Read the model definition and answer for the solid it produces. Units are mm, in the model's axes. Face numbers are marked on the shaded views. A direction names the side the tool comes from. Coordinates: 2 decimals unless noted, no trailing zeros. Order: outer loops, then holes, each group sorted by start corner. A loop starts at its lowest first (then second) coordinate and runs counter-clockwise, first axis right, second up. Notation, with made-up numbers: (-31, -10) - (1, -10) arc R12 ccw to (1, -6) - close; hole circle Ø11 at (-0.5, -14.75). An arc over 180 degrees is marked (long way). Use one line per item in the form item = value.
```python
from build123d import *

# Parameters (mm, degrees)
SKETCH_1_R             = 11
SKETCH_1_R_2           = 1.75
EXTRUDE_1_DEPTH        = 3.6
SKETCH_2_R             = 5
SKETCH_2_R_2           = 4
EXTRUDE_1_2_DEPTH      = 10
EXTRUDE_1_2_DEPTH_BACK = 5.1
SKETCH_3_R             = 4
CUT_EXTRUDE_1_DEPTH    = 14.6


with BuildPart() as part:
    # Эскиз1 → Extrude 1 (new body)
    with BuildSketch(Plane.XY):
        Circle(SKETCH_1_R)
        with Locations((0, 8)):
            Circle(SKETCH_1_R_2, mode=Mode.SUBTRACT)
        with Locations((8, 0)):
            Circle(SKETCH_1_R_2, mode=Mode.SUBTRACT)
        with Locations((0, -8)):
            Circle(SKETCH_1_R_2, mode=Mode.SUBTRACT)
        with Locations((-8, 0)):
            Circle(SKETCH_1_R_2, mode=Mode.SUBTRACT)
    extrude(amount=EXTRUDE_1_DEPTH)

    # Эскиз2 → Extrude 1 2 (add, two sides)
    with BuildSketch(Plane.XY.offset(3.6)) as extrude_1_2_sk:
        Circle(SKETCH_2_R)
        Circle(SKETCH_2_R_2, mode=Mode.SUBTRACT)
    extrude(amount=EXTRUDE_1_2_DEPTH)
    extrude(extrude_1_2_sk.sketch, amount=-EXTRUDE_1_2_DEPTH_BACK)

    # Эскиз3 → Вырез-Вытянуть1 (cut, through all)
    with BuildSketch(Plane(origin=(0, 0, 0), x_dir=(-1, 0, 0), z_dir=(0, 0, -1))):
        Circle(SKETCH_3_R)
    extrude(amount=-CUT_EXTRUDE_1_DEPTH, mode=Mode.SUBTRACT)


solid = part.part
```
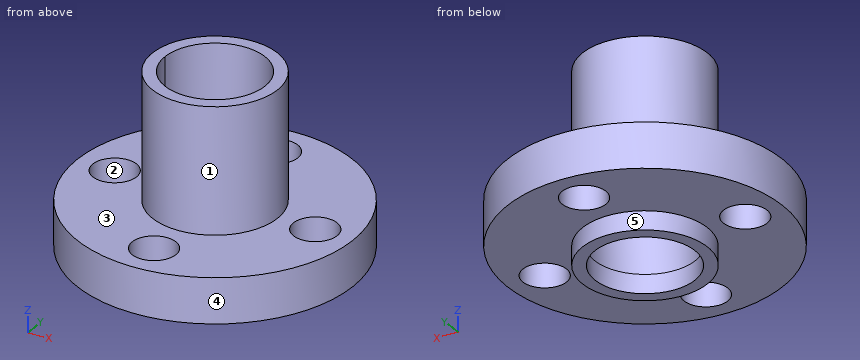
(1) Given pin 1 Ø3 at (x, y) = (8.5, 0.5) entering from +Z; pin 2 Ø1.5 at (x, z) = (1, 3.5) entering from +Y; pin 3 Ø3 at (x, z) = (-7.5, 4) entering from -Y, each flat-ended and moving along its own axis, determine where each tip first touches the part or whether it passes through.
Answer list:
pin_1 = 3.6
pin_2 = 11
pin_3 = -9.18
(2) Section A-A, the plane x = 0 is taken. Write down the section's boundary in (y, z), then the cut area to 3 significant figures.
Answer list:
outline = (-11, 0) - (-9.75, 0) - (-9.75, 3.6) - (-11, 3.6) - close; (-6.25, 0) - (-5, 0) - (-5, -1.5) - (-4, -1.5) - (-4, 13.6) - (-5, 13.6) - (-5, 3.6) - (-6.25, 3.6) - close; (4, -1.5) - (5, -1.5) - (5, 0) - (6.25, 0) - (6.25, 3.6) - (5, 3.6) - (5, 13.6) - (4, 13.6) - close; (9.75, 0) - (11, 0) - (11, 3.6) - (9.75, 3.6) - close
area = 48.2 mm2
(3) Section C-C, the plane y = -8.5 is taken. Write down the section's boundary in (x, z), then the cut area to 3 significant figures.
Answer list:
outline = (-6.98, 0) - (-1.68, 0) - (-1.68, 3.6) - (-6.98, 3.6) - close; (1.68, 0) - (6.98, 0) - (6.98, 3.6) - (1.68, 3.6) - close
area = 38.2 mm2
(4) Straight lines are drawn through the part: L1, parallel to Y at x = 0, z = 1.4; L2, parallel to Y at x = 0, z = -1.1; L3, parallel to X at y = -2, z = 8.25. For each, find the intervals that lie inside material, in ascending order.
Answer list:
L1 = -11 to -9.75, -6.25 to -4, 4 to 6.25, 9.75 to 11
L2 = -5 to -4, 4 to 5
L3 = -4.58 to -3.46, 3.46 to 4.58
(5) Which of the six approach directions +Z, -Z, +X, -X, +Y, -Y give full straight-line access (tool end or side, diameter ignored) to the marked faces 4 and 5?
Answer list:
face_4 = +Z, -Z
face_5 = -Z
(6) Section B-B, the plane z = 6.75 is taken. Write down the section's boundary in (x, y).
Answer list:
outline = circle Ø10 at (0, 0); hole circle Ø8 at (0, 0)
(7) Section D-D, the plane x = -8 is taken. Write down the section's boundary in (y, z), then the cut area to 3 significant figures.
Answer list:
outline = (-7.55, 0) - (-1.75, 0) - (-1.75, 3.6) - (-7.55, 3.6) - close; (1.75, 0) - (7.55, 0) - (7.55, 3.6) - (1.75, 3.6) - close
area = 41.8 mm2
(8) The mould has two halves that part along Y. Classify the marked faces 1, 2 and 3: +Y half, -Y half, draft (parallel to the pull), parting line (faces both ways), or undercut.
Answer list:
face_1 = parting line
face_2 = undercut
face_3 = draft
